Geometry check sheet. Reference: the model listing, model coordinates, mm. Face numbers are marked on the shaded views. A direction names the side the tool comes from. Coordinates: 2 decimals unless noted, no trailing zeros. Loops run counter-clockwise (first coordinate to the right, second up) from the corner with the lowest first, then second, coordinate; pieces in that order, holes last.
from build123d import *

# Parameters (mm, degrees)
SKETCH_1_W      = 62.3
SKETCH_1_H      = 34.3
EXTRUDE_1_DEPTH = 10.6
SKETCH_1_3_W    = 62.3
SKETCH_1_3_H    = 10
EXTRUDE_2_DEPTH = 12.6
SKETCH_4_R      = 9.593725323
EXTRUDE_3_DEPTH = 23.62
FILLET_1_R      = 5


with BuildPart() as part:
    # Sketch 1 → Extrude 1 (new body)
    with BuildSketch(Plane(origin=(0, 0, 0), x_dir=(1, 0, 0), z_dir=(0, 1, 0))):
        with Locations((0, 5)):
            Rectangle(SKETCH_1_W, SKETCH_1_H)
    extrude(amount=EXTRUDE_1_DEPTH)

    # Sketch 1_3 → Extrude 2 (add)
    with BuildSketch(Plane(origin=(0, 0, 0), x_dir=(1, 0, 0), z_dir=(0, 1, 0))):
        with Locations((0, -17.15)):
            Rectangle(SKETCH_1_3_W, SKETCH_1_3_H)
    extrude(amount=EXTRUDE_2_DEPTH)

    # Sketch 4 → Extrude 3 (add)
    with BuildSketch(Plane(origin=(0, 10.6, 0), x_dir=(1, 0, 0), z_dir=(0, 1, 0))):
        with Locations(Location((0, 5.500207834, 0), (0, 0, 270))):
            Circle(SKETCH_4_R)
    extrude(amount=EXTRUDE_3_DEPTH)

    # Fillet 1
    fillet_1_edges = [part.edges().sort_by_distance(p)[0] for p in [
        (31.15, 6.3, 22.15),
        (-31.15, 6.3, 22.15),
        (-31.15, 5.3, -22.15),
        (31.15, 5.3, -22.15),
    ]]
    fillet(fillet_1_edges, radius=FILLET_1_R)


solid = part.part
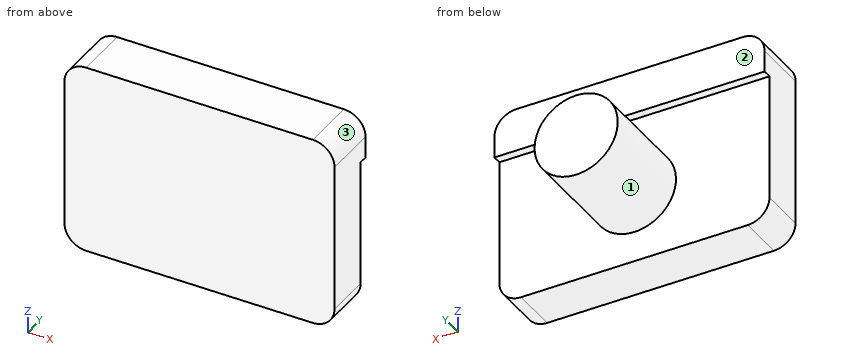
(1) Sectioned sample at C-C on y = 23. Record the cut outline in (x, z), and give its area (3 significant figures).
Findings:
outline: circle Ø19.19 at (0, -5.5)
area: 289 mm2
(2) Scan lines: L1, parallel to Y at x = -27, z = -15.5; L2, parallel to Y at x = -19, z = 19.5; L3, parallel to X at y = 25, z = -6. Record each from-to range of solid material in increasing order.
Findings:
L1: y = 0 to 10.6
L2: y = 0 to 12.6
L3: x = -9.58 to 9.58
(3) Sectioned sample at D-D on x = 13.5. Record the cut outline in (y, z).
Findings:
outline: (0, -22.15) - (10.6, -22.15) - (10.6, 12.15) - (12.6, 12.15) - (12.6, 22.15) - (0, 22.15) - close
(4) Sectioned sample at B-B on z = -3. Record the cut outline in (x, y).
Findings:
outline: (-31.15, 0) - (31.15, 0) - (31.15, 10.6) - (9.26, 10.6) - (9.26, 34.22) - (-9.26, 34.22) - (-9.26, 10.6) - (-31.15, 10.6) - close
(5) Sectioned sample at A-A on x = 0. Record the cut outline in (y, z), and give its area (3 significant figures).
Findings:
outline: (0, -22.15) - (10.6, -22.15) - (10.6, -15.09) - (34.22, -15.09) - (34.22, 4.09) - (10.6, 4.09) - (10.6, 12.15) - (12.6, 12.15) - (12.6, 22.15) - (0, 22.15) - close
area: 943 mm2
(6) Access from +Z, -Z, +X, -X, +Y, -Y to the whole of each face (thin tool, end or side, straight path). Record for the marked faces 1, 2 and 3.
Findings:
face 1: +Y
face 2: +Z, +X, -X, +Y
face 3: +Z, +X, +Y, -Y
(7) Gauge pin test, flat ends, axial feed: pin 1 Ø5 at (y, z) = (22, 3.5) entering from -X; pin 2 Ø8 at (x, z) = (-1.5, 10.5) entering from +Y; pin 3 Ø5 at (y, z) = (25.5, -2.5) entering from -X; pin 4 Ø12 at (x, z) = (-16.5, -12.5) entering from -Y. Record the tip position at first contact, or that the pin passes through.
Findings:
pin 1: stops at x = -7.06
pin 2: stops at y = 12.6
pin 3: stops at x = -9.58
pin 4: stops at y = 0
